For this review, use the dimensioned drawing (mm, ordinates from the lowest corner) and the shaded views. Round coordinates to 2 decimals unless told otherwise and drop trailing zeros. Order: outer loops, then holes, each group sorted by start corner. A loop starts at its lowest first (then second) coordinate and runs counter-clockwise, first axis right, second up. Notation, with made-up numbers: (-4.75, 58) -> (34.25, 58) arc R22 cw to (34.25, 85) -> close; hole circle Ø3 at (0.5, 23.5). An arc over 180 degrees is marked (long way). Answer in a Markdown table with one row per item.
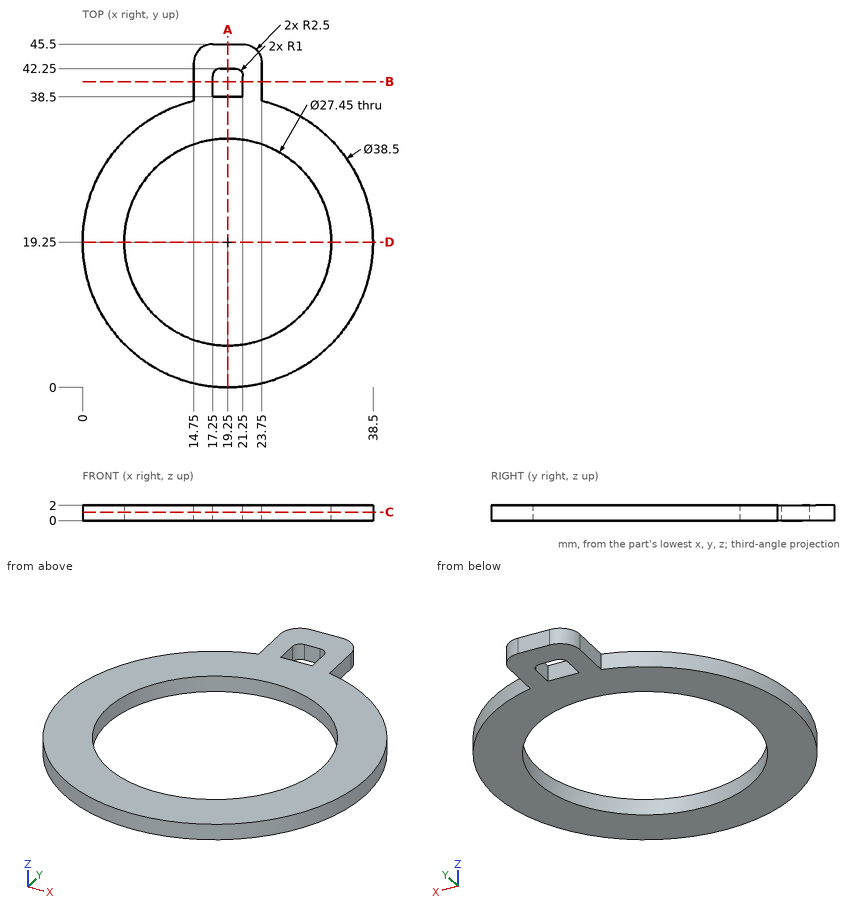
Q1. Take a section at D-D, the plane y = 19.25. Write out the cut boundary in (x, z) (3 decimals), then the cut area to 3 significant figures.
Answer key:
| item | result |
|---|---|
| outline | (0, 0) -> (5.525, 0) -> (5.525, 2) -> (0, 2) -> close; (32.975, 0) -> (38.5, 0) -> (38.5, 2) -> (32.975, 2) -> close |
| area | 22.1 mm^2 |
Q2. Take a section at B-B, the plane y = 40.5. Write out the cut boundary in (x, z).
Answer key:
| item | result |
|---|---|
| outline | (14.75, 0) -> (17.25, 0) -> (17.25, 2) -> (14.75, 2) -> close; (21.25, 0) -> (23.75, 0) -> (23.75, 2) -> (21.25, 2) -> close |
Q3. To check wall thickness, follow probe 1 along Y at (x, z) = (19.25, 0.55) (3 decimals); probe 2 along X at (y, z) = (19.25, 0.55) (3 decimals); probe 3 along Y at (x, z) = (18, 1.9). State the ranges of each line that lie inside material, in increasing order.
Answer key:
| item | result |
|---|---|
| probe 1 | y = 0 to 5.525, 32.975 to 38.5, 42.25 to 45.5 |
| probe 2 | x = 0 to 5.525, 32.975 to 38.5 |
| probe 3 | y = 0.04 to 5.58, 32.92 to 38.5, 42.22 to 45.5 |
Q4. Take a section at C-C, the plane z = 1.1. Write out the cut boundary in (x, y) (3 decimals).
Answer key:
| item | result |
|---|---|
| outline | (14.75, 37.967) arc R19.25 ccw (long way) to (23.75, 37.967) -> (23.75, 43) arc R2.5 ccw to (21.25, 45.5) -> (17.25, 45.5) arc R2.5 ccw to (14.75, 43) -> close; hole circle Ø27.45 at (19.25, 19.25); hole (17.25, 38.5) -> (21.25, 38.5) -> (21.25, 41.25) arc R1 ccw to (20.25, 42.25) -> (18.25, 42.25) arc R1 ccw to (17.25, 41.25) -> close |
Q5. Clearance check with flat-ended pins moving along their axes: pin 1 Ø1 at (y, z) = (39.5, 0.5) entering from -X; pin 2 Ø0.6 at (y, z) = (40, 1) entering from +X. State where each tip first meets the part, or that it passes through.
Answer key:
| item | result |
|---|---|
| pin 1 | stops at x = 14.75 |
| pin 2 | stops at x = 23.75 |
Q6. Take a section at A-A, the plane x = 19.25. Write out the cut boundary in (y, z) (3 decimals), then the cut area to 3 significant figures.
Answer key:
| item | result |
|---|---|
| outline | (0, 0) -> (5.525, 0) -> (5.525, 2) -> (0, 2) -> close; (32.975, 0) -> (38.5, 0) -> (38.5, 2) -> (32.975, 2) -> close; (42.25, 0) -> (45.5, 0) -> (45.5, 2) -> (42.25, 2) -> close |
| area | 28.6 mm^2 |
